from build123d import *

# Parameters (mm, degrees)
SKETCH1_R                    = 2.475
BOSS_EXTRUDE1_DEPTH          = 25.2
SKETCH2_R                    = 5
BOSS_EXTRUDE2_DEPTH          = 3
M2_5X0_45_TAPPED_HOLE2_D     = 2.05
M2_5X0_45_TAPPED_HOLE2_DEPTH = 7.25
M2_5X0_45_TAPPED_HOLE2_TIP   = 0.615882135
CUT_EXTRUDE1_DEPTH           = 1


with BuildPart() as part:
    # Sketch1 → Boss-Extrude1 (new body)
    with BuildSketch(Plane(origin=(0, 0, 0), x_dir=(1, 0, 0), z_dir=(0, 1, 0))):
        with Locations(Location((0, 0, 0), (0, 0, 270))):
            Circle(SKETCH1_R)
    extrude(amount=BOSS_EXTRUDE1_DEPTH)

    # Sketch2 → Boss-Extrude2 (add)
    with BuildSketch(Plane(origin=(0, 25.2, 0), x_dir=(1, 0, 0), z_dir=(0, 1, 0))):
        with Locations(Location((0, 0, 0), (0, 0, 270))):
            Circle(SKETCH2_R)
    extrude(amount=BOSS_EXTRUDE2_DEPTH)

    # M2.5x0.45 Tapped Hole2
    with Locations(Plane(origin=(0, 0, 0), x_dir=(-1, 0, 0), z_dir=(0, -1, 0))):
        with Locations((0, 0)):
            Hole(M2_5X0_45_TAPPED_HOLE2_D / 2, depth=M2_5X0_45_TAPPED_HOLE2_DEPTH)
            with Locations((0, 0, -(M2_5X0_45_TAPPED_HOLE2_DEPTH + M2_5X0_45_TAPPED_HOLE2_TIP / 2))):  # 118° drill point
                Cone(0, M2_5X0_45_TAPPED_HOLE2_D / 2, M2_5X0_45_TAPPED_HOLE2_TIP, mode=Mode.SUBTRACT)

    # Sketch15 → Cut-Extrude1 (cut)
    with BuildSketch(Plane(origin=(0, 28.2, 0), x_dir=(1, 0, 0), z_dir=(0, 1, 0))):
        Polygon((-0.96474359, 1.812951114), (1.233974359, 1.812951114), (1.233974359, 1.453976755), (-0.516025641, 1.453976755), (-0.516025641, 0.377053678), (1.233974359, 0.377053678), (1.233974359, 0.018079319), (-0.516025641, 0.018079319), (-0.516025641, -1.687048886), (-0.96474359, -1.687048886), align=None)
    extrude(amount=-CUT_EXTRUDE1_DEPTH, mode=Mode.SUBTRACT)


solid = part.part
The listing builds one solid part. Answer for the finished solid, in the listing's coordinates (mm). A direction names the side the tool comes from. Coordinates: 2 decimals unless noted, no trailing zeros. Order: outer loops, then holes, each group sorted by start corner. A loop starts at its lowest first (then second) coordinate and runs counter-clockwise, first axis right, second up. Notation, with made-up numbers: (46, 59.25) -> (99, 59.25) arc R21 ccw to (99, 96.25) -> close; hole circle Ø2 at (-2, -23). An arc over 180 degrees is marked (long way). Answer in a Markdown table with one row per item. Add a question column.
Item 1: Which of the six approach directions +Z, -Z, +X, -X, +Y, -Y give full straight-line access (tool end or side, diameter ignored) to faces 4 (the face through (0, 28, -1.813)), 5 (the face through (-0.133, 3.676, -1.016)), 6 (the face through (0, 28.2, 1))?
Item 2: Determine the mould class of faces 1 (the face through (0, 28, -0.018)), 2 (the face through (0.74, 12.42, 2.36)), 3 (the face through (-1, 0, 1)) for opening direction Z: +Z half, -Z half, draft (parallel to the pull), parting line (faces both ways), or undercut.
Item 3: Find section D-D (y = 21.75). Write down the section's boundary in (x, z) (3 decimals).
Item 4: Find section A-A (y = 6). Write down the section's boundary in (x, z) (3 decimals), then the cut area to 3 significant figures.
Item 5: Find section B-B (x = 3). Write down the section's boundary in (y, z), then the cut area to 3 significant figures.
Item 6: Find the intervals of material crossed by L1, parallel to Y at x = 4, z = 0.25; L2, parallel to X at y = 19, z = 2.25; L3, parallel to X at y = 23, z = -2, in increasing order. Write a range as from..to.
Item 7: Each of these flat-tipped pins is pushed along its axis until it touches: P1, Ø4, axis at y = 21, z = -3, coming from the -X side; P2, Ø6, axis at y = 21, z = 3, coming from the +X side (3 decimals); P3, Ø4, axis at y = 17.5, z = -3, coming from the +X side. Where does it stop, or does it pass through?
Item 8: Find section C-C (z = -3). Write down the section's boundary in (x, y), then the cut area to 3 significant figures.
Result set:
| question | item | result |
|---|---|---|
| 1 | face 4 | +Y |
| 1 | face 5 | -Y |
| 1 | face 6 | +Z, -Z, +X, -X, +Y |
| 2 | face 1 | undercut |
| 2 | face 2 | parting line |
| 2 | face 3 | draft |
| 3 | outline | circle Ø4.95 at (0, 0) |
| 4 | outline | circle Ø4.95 at (0, 0); hole circle Ø2.05 at (0, 0) |
| 4 | area | 15.9 mm² |
| 5 | outline | (25.2, -4) -> (28.2, -4) -> (28.2, 4) -> (25.2, 4) -> close |
| 5 | area | 24.0 mm² |
| 6 | L1 | y = 25.2..28.2 |
| 6 | L2 | x = -1.03..1.03 |
| 6 | L3 | x = -1.46..1.46 |
| 7 | P1 | stops at x = -2.26 |
| 7 | P2 | stops at x = 2.475 |
| 7 | P3 | stops at x = 2.26 |
| 8 | outline | (-4, 25.2) -> (4, 25.2) -> (4, 28.2) -> (-4, 28.2) -> close |
| 8 | area | 24.0 mm² |
